Read the model definition and answer for the solid it produces. Units are mm, in the model's axes. Face numbers are marked on the shaded views. A direction names the side the tool comes from. Give positions to 0.01 mm unless a question says otherwise; leave off trailing zeros. Order: outer loops, then holes, each group sorted by start corner. A loop starts at its lowest first (then second) coordinate and runs counter-clockwise, first axis right, second up. Notation, with made-up numbers: (2.5, 34) - (47.5, 34) arc R20 ccw to (47.5, 51) - close; hole circle Ø4 at (55, 14.25). An arc over 180 degrees is marked (long way). Use a Markdown table: item, result. Add a question column.
1. A cutting plane is placed at A-A on x = -18. Determine the outline of the cut face in (y, z), and give its area (3 significant figures).
2. For a pull along Y with two mould halves and no side action, classify the marked faces 5, 6, 7 and 8 as released by +Y, released by -Y, zero draft, split by the parting line, or undercut.
3. A cutting plane is placed at B-B on y = 16. Determine the outline of the cut face in (x, z).
4. A cutting plane is placed at C-C on x = -7.5. State how many separate pieces and enclosed holes the cut face has, and give its area (3 significant figures).
5. A cutting plane is placed at D-D on y = -11. Determine the outline of the cut face in (x, z), and give its area (3 significant figures).
6. Consider L1, parallel to X at y = 16, z = 4; L2, parallel to Y at x = -18, z = 6; L3, parallel to X at y = 0.5, z = 13. Determine where each line is inside the solid, lowest interval first.
7. Flat-ended cylindrical pins translate along their axes: P1, Ø13, axis at y = 10.61, z = 33.54, coming from the +X side; P2, Ø11, axis at y = 3, z = 23, coming from the -X side; P3, Ø6, axis at y = -3.54, z = 19.39, coming from the +X side; P4, Ø5, axis at x = -18, y = -16, coming from the -Z side. Find the tip coordinate at first contact, or state that the pin passes through.
8. Which of the six approach directions +Z, -Z, +X, -X, +Y, -Y give full straight-line access (tool end or side, diameter ignored) to the marked faces 1, 2, 3 and 4?
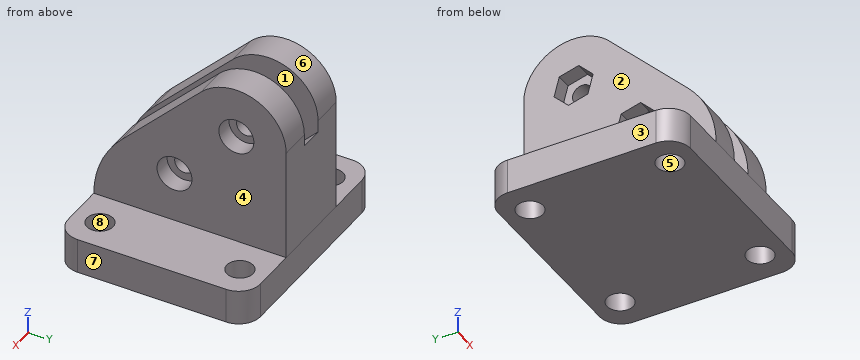
Solid Edge part; units mm, degrees
sketch "Sketch1" plane through (0, 0, 0) normal (0, 0, 1) x (1, 0, 0)
  line L0 (25.25, -22) -> (25.25, 22)
  line L1 (25.25, 22) -> (-25.25, 22)
  line L2 (-25.25, 22) -> (-25.25, -22)
  line L3 (-25.25, -22) -> (25.25, -22)
extrude "Protrusion1" add sketch "Sketch1" along normal blind 8
sketch "Sketch2" plane through (0, 0, 0) normal (1, 0, 0) x (0, 1, 0)
  line L0 (22, 33.5355) -> (22, 8)
  line L1 (22, 8) -> (-22, 8)
  arc A0 (-15.5565, 23.4852) -> (-22, 8) centre (-0.0001, 7.9288) ccw
  line L2 (2.5503, 41.5919) -> (-15.5565, 23.4852)
  arc A1 (2.5503, 41.5919) -> (22, 33.5355) centre (10.6066, 33.5355) cw
extrude "ProtrusiónExtruida_2" add sketch "Sketch2" along normal mid plane 20
sketch "Sketch3" plane through (0, 0, 0) normal (1, 0, 0) x (0, 1, 0)
  line L0 (-0.7868, 8) -> (22, 30.7868)
  line L1 (22, 30.7868) -> (22, 33.5355)
  line L2 (2.5503, 41.5919) -> (-15.5565, 23.4852)
  arc A0 (-15.5565, 23.4852) -> (-22, 8) centre (-0.0001, 7.9288) ccw
  line L3 (-0.7868, 8) -> (-22, 8)
  arc A1 (2.5503, 41.5919) -> (22, 33.5355) centre (10.6066, 33.5355) cw
extrude "VaciadoExtruido_1" cut sketch "Sketch3" along normal mid plane 5.5
hole "Agujero_1" at (10, 10.6066, 33.5355) direction (-1, 0, 0) diameter 4.5 end through all counterbore diameter 8 counterbore depth 4
hole "Hole1" at (10, -3.5355, 19.3934) direction (-1, 0, 0) diameter 4.5 end through all counterbore diameter 8 counterbore depth 4
sketch "Sketch4" plane through (-10, 0, 26.4645) normal (-1, 0, 0) x (0, -1, 0)
  line L0 (-6.1452, 8.2665) -> (-9.4112, 11.5325)
  line L1 (-9.4112, 11.5325) -> (-13.8726, 10.3371)
  line L2 (-13.8726, 10.3371) -> (-15.068, 5.8756)
  line L3 (-15.068, 5.8756) -> (-11.802, 2.6096)
  line L4 (-11.802, 2.6096) -> (-7.3406, 3.8051)
  line L5 (-7.3406, 3.8051) -> (-6.1452, 8.2665)
  line L6 (7.997, -5.8756) -> (4.731, -2.6096)
  line L7 (4.731, -2.6096) -> (0.2695, -3.8051)
  line L8 (0.2695, -3.8051) -> (-0.9259, -8.2665)
  line L9 (-0.9259, -8.2665) -> (2.3401, -11.5325)
  line L10 (2.3401, -11.5325) -> (6.8015, -10.3371)
  line L11 (6.8015, -10.3371) -> (7.997, -5.8756)
extrude "VaciadoExtruido_2" cut sketch "Sketch4" against normal blind 3.5
hole "Agujero_3" at (18, 16, 8) direction (0, 0, -1) diameter 6 end through all
hole "Hole2" at (18, -16, 8) direction (0, 0, -1) diameter 6 end through all
hole "Hole3" at (-18, -16, 8) direction (0, 0, -1) diameter 6 end through all
hole "Hole4" at (-18, 16, 8) direction (0, 0, -1) diameter 6 end through all
fillet "Redondeo_1" radius 5 4 edges at (25.25, -22, 4) (-25.25, -22, 4) (-25.25, 22, 4) (25.25, 22, 4)
Output values:
| question | item | result |
|---|---|---|
| 1 | outline | (-22, 0) - (-19, 0) - (-19, 8) - (-22, 8) - close; (-13, 0) - (13, 0) - (13, 8) - (-13, 8) - close; (19, 0) - (22, 0) - (22, 8) - (19, 8) - close |
| 1 | area | 256 mm² |
| 2 | face 5 | undercut |
| 2 | face 6 | split by the parting line |
| 2 | face 7 | zero draft |
| 2 | face 8 | undercut |
| 3 | outline | (-25.25, 0) - (-21, 0) - (-21, 8) - (-25.25, 8) - close; (-15, 0) - (15, 0) - (15, 8) - (10, 8) - (10, 43.57) - (2.75, 43.57) - (2.75, 24.79) - (-2.75, 24.79) - (-2.75, 43.57) - (-10, 43.57) - (-10, 8) - (-15, 8) - close; (21, 0) - (25.25, 0) - (25.25, 8) - (21, 8) - close |
| 4 | separate pieces | 1 |
| 4 | enclosed holes | 2 |
| 4 | area | 1,440 mm² |
| 5 | outline | (-25.25, 0) - (25.25, 0) - (25.25, 8) - (10, 8) - (10, 28.04) - (2.75, 28.04) - (2.75, 8) - (-2.75, 8) - (-2.75, 28.04) - (-10, 28.04) - (-10, 8) - (-25.25, 8) - close |
| 5 | area | 695 mm² |
| 6 | L1 | -25.25 to -21, -15 to 15, 21 to 25.25 |
| 6 | L2 | -22 to -19, -13 to 13, 19 to 22 |
| 6 | L3 | -10 to -2.75, 2.75 to 10 |
| 7 | P1 | x = 10 |
| 7 | P2 | x = -10 |
| 7 | P3 | x = 6 |
| 7 | P4 | through |
| 8 | face 1 | +Z, -Y |
| 8 | face 2 | +Z, -X, +Y, -Y |
| 8 | face 3 | +Z, -Z, -X, +Y, -Y |
| 8 | face 4 | +Z, +X, +Y, -Y |
